The drawing under review shows one solid part. Ordinate dimensions are in mm from its lowest x, y, z. A direction names the side the tool comes from. Give positions to 0.01 mm unless a question says otherwise; leave off trailing zeros. Order: outer loops, then holes, each group sorted by start corner. A loop starts at its lowest first (then second) coordinate and runs counter-clockwise, first axis right, second up. Notation, with made-up numbers: (88, 3) -> (145, 3) arc R18 ccw to (145, 32) -> close; hole circle Ø9 at (35.5, -31.75). An arc over 180 degrees is marked (long way). Return JSON: item names as keys, results as strings. Group by question number.
1) Add section C-C (z = 36). Give the boundary of the cut face in (x, y), then the cut area to 3 significant figures.
2) Add section D-D (z = 15.5). Give the boundary of the cut face in (x, y), then the cut area to 3 significant figures.
3) Add section B-B (y = 15). Give the boundary of the cut face in (x, z).
4) The part is to be moulded in two halves that separate along Y. For the marked faces 4, 5, 6 and 7, say which applies: released by +Y, released by -Y, zero draft, split by the parting line, or undercut.
5) For the marked faces 1, 2 and 3, list the 3-axis set-ups (+Z, -Z, +X, -X, +Y, -Y) from which the entire face can be reached by the end or side of a thin tool; tool diameter is ignored.
6) Add section A-A (y = 31). Give the boundary of the cut face in (x, z), then the cut area to 3 significant figures.
7) Insertion check: P1, Ø4, axis at x = 20.5, y = 62.5, coming from the -Z side; P2, Ø2, axis at x = 24, z = 14, coming from the -Y side; P3, Ø4, axis at x = 21, z = 12, coming from the +Y side. Each pin has a flat end and moves straight along its axis. Give the tip position at first contact, or say it passes through.
8) To check wall thickness, follow line 1 along X through (y, z) = (41, 31); line 2 along Y through (x, z) = (76, 20.5); line 3 along Z through (x, y) = (7, 15). State the ranges of each line that lie inside material, in increasing order.
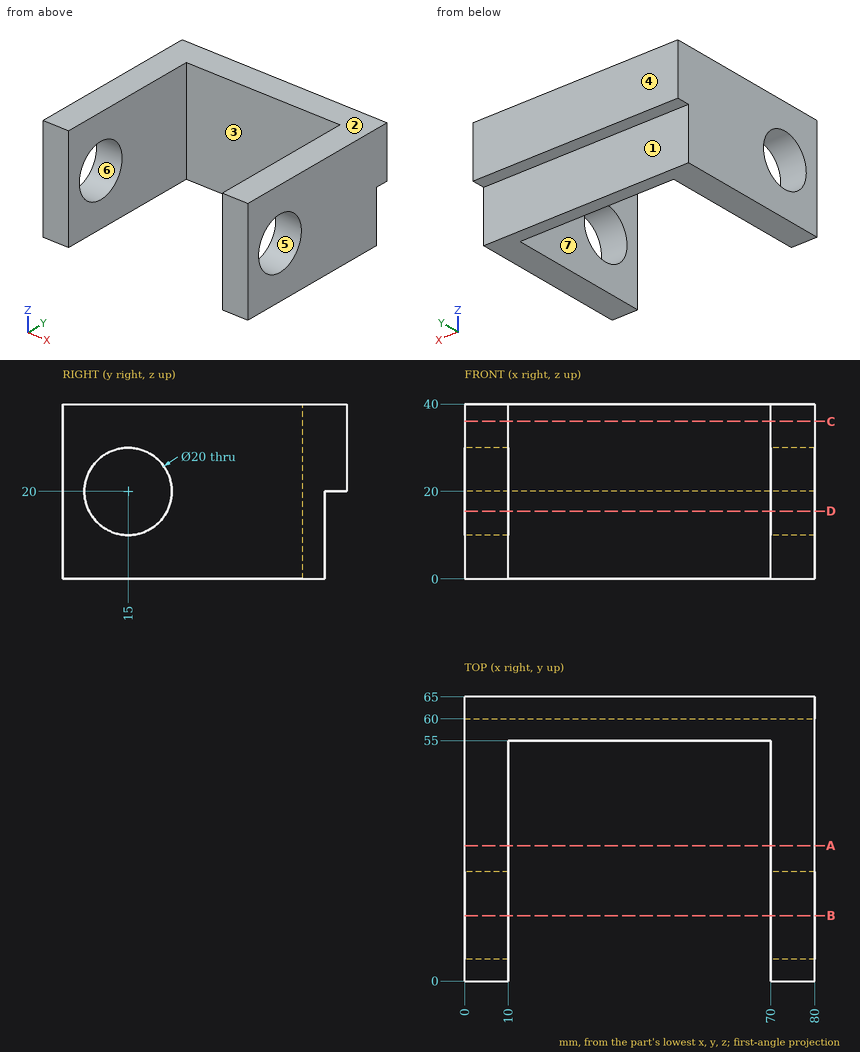
Evaluation:
{
 "1": {"outline": "(0, 0) -> (10, 0) -> (10, 55) -> (70, 55) -> (70, 0) -> (80, 0) -> (80, 65) -> (0, 65) -> close", "area": "1,900 mm^2"},
 "2": {"outline": "(0, 0) -> (10, 0) -> (10, 6.07) -> (0, 6.07) -> close; (0, 23.93) -> (10, 23.93) -> (10, 55) -> (70, 55) -> (70, 23.93) -> (80, 23.93) -> (80, 60) -> (0, 60) -> close; (70, 0) -> (80, 0) -> (80, 6.07) -> (70, 6.07) -> close", "area": "1,140 mm^2"},
 "3": {"outline": "(0, 0) -> (10, 0) -> (10, 10) -> (0, 10) -> close; (0, 30) -> (10, 30) -> (10, 40) -> (0, 40) -> close; (70, 0) -> (80, 0) -> (80, 10) -> (70, 10) -> close; (70, 30) -> (80, 30) -> (80, 40) -> (70, 40) -> close"},
 "4": {"face 4": "released by +Y", "face 5": "undercut", "face 6": "undercut", "face 7": "zero draft"},
 "5": {"face 1": "-Z, +X, -X, +Y", "face 2": "+Z, +X, -X, +Y, -Y", "face 3": "+Z, -Z, -Y"},
 "6": {"outline": "(0, 0) -> (10, 0) -> (10, 40) -> (0, 40) -> close; (70, 0) -> (80, 0) -> (80, 40) -> (70, 40) -> close", "area": "800 mm^2"},
 "7": {"P1": "z = 20", "P2": "y = 55", "P3": "y = 60"},
 "8": {"line 1": "0 to 10, 70 to 80", "line 2": "0 to 5.01, 24.99 to 65", "line 3": "0 to 10, 30 to 40"}
}
